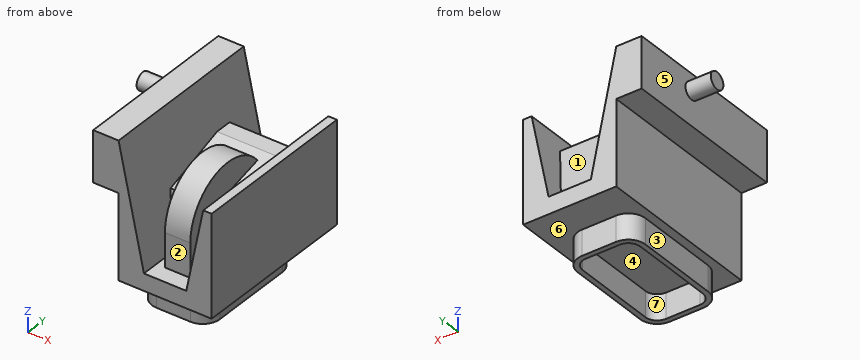
from build123d import *

# Parameters (mm, degrees)
F1_DEPTH      = 100
F4_DEPTH      = 20.5
F4_DEPTH_BACK = 21.0714285714
F6_DEPTH      = 7.5
F6_DEPTH_BACK = 7.5
F7_W          = 15
F7_H          = 30
F8_DEPTH      = 100
F9_R          = 5
F10_DEPTH     = 15
F11_W         = 40
F11_H         = 70
F12_DEPTH     = 15
F13_R         = 10
F15_DEPTH     = 15


with BuildPart() as f1:
    # F0 (on Front) → F1 (new body)
    with BuildSketch(Plane.XZ):
        Polygon((15, 10), (0, 80), (0, 0), (55, 0), (55, 60), (50, 60), (40, 10), align=None)
    extrude(amount=-F1_DEPTH)

    # F3 (on offset) → F4 (join, two sides)
    with BuildSketch(Plane.YZ.offset(27.5)) as f4_sk:
        Polygon((30, 40), (21.9615242271, 10), (90, 10), (80, 50), (70, 50), align=None)
    extrude(amount=F4_DEPTH)
    extrude(f4_sk.sketch, amount=-F4_DEPTH_BACK)

    # F5 (on offset) → F6 (join, two sides)
    with BuildSketch(Plane.YZ.offset(27.5)) as f6_sk:
        with BuildLine():
            Line((10, 0), (40, 0))
            ThreePointArc((40, 0), (61.2132034356, 51.2132034356), (10, 30))
            Line((10, 30), (10, 0))
        make_face()
    extrude(amount=F6_DEPTH)
    extrude(f6_sk.sketch, amount=-F6_DEPTH_BACK)

    # F7 (on face) → F8 (join)
    with BuildSketch(Plane.XZ):
        with Locations((-7.5, 65)):
            Rectangle(F7_W, F7_H)
    extrude(amount=-F8_DEPTH)

    # F9 (on face) → F10 (join)
    with BuildSketch(Plane(origin=(-15, 0, 0), x_dir=(0, -1, 0), z_dir=(-1, 0, 0))):
        with Locations((-60, 70)):
            Circle(F9_R)
    extrude(amount=F10_DEPTH)

    # F11 (on face) → F12 (join)
    with BuildSketch(Plane(origin=(0, 0, 0), x_dir=(1, 0, 0), z_dir=(0, 0, -1))):
        with Locations((25, -45)):
            Rectangle(F11_W, F11_H)
    extrude(amount=F12_DEPTH)

    # F13
    f13_edges = [f1.edges().sort_by_distance(p)[0] for p in [
        (45, 10, -7.5),
        (5, 10, -7.5),
        (45, 80, -7.5),
        (5, 80, -7.5),
    ]]
    fillet(f13_edges, radius=F13_R)

    # F14 (on face) → F15 (cut)
    with BuildSketch(Plane(origin=(0, 0, -15), x_dir=(1, 0, 0), z_dir=(0, 0, -1))):
        with BuildLine():
            Line((8, -20), (8, -70))
            ThreePointArc((8, -70), (10.0502525317, -74.9497474683), (15, -77))
            Line((15, -77), (35, -77))
            ThreePointArc((35, -77), (39.9497474683, -74.9497474683), (42, -70))
            Line((42, -70), (42, -20))
            ThreePointArc((42, -20), (39.9497474683, -15.0502525317), (35, -13))
            Line((35, -13), (15, -13))
            ThreePointArc((15, -13), (10.0502525317, -15.0502525317), (8, -20))
        make_face()
    extrude(amount=-F15_DEPTH, mode=Mode.SUBTRACT)


solid = f1.part
The model under review builds one solid part; all positions refer to its coordinate system, in mm. Face numbers are marked on the shaded views. A direction names the side the tool comes from. Round coordinates to 2 decimals unless told otherwise and drop trailing zeros. Order: outer loops, then holes, each group sorted by start corner. A loop starts at its lowest first (then second) coordinate and runs counter-clockwise, first axis right, second up. Notation, with made-up numbers: (70, 72.5) -> (83, 72.5) arc R10 ccw to (83, 77.5) -> close; hole circle Ø7 at (-24.75, -7). An arc over 180 degrees is marked (long way). Return JSON: item names as keys, results as strings.
1. Insertion check: P1, Ø15, axis at y = 49, z = 19, coming from the -X side; P2, Ø16.5, axis at x = 27, y = 52, coming from the -Z side; P3, Ø16.5, axis at x = 25.5, z = -8.5, coming from the +Y side. Each pin has a flat end and moves straight along its axis. Give the tip position at first contact, or say it passes through.
Answer block:
{"P1": "stops at x = 0", "P2": "stops at z = 0", "P3": "stops at y = 80"}
2. For the marked faces 1, 2, 3 and 4, list the 3-axis set-ups (+Z, -Z, +X, -X, +Y, -Y) from which the entire face can be reached by the end or side of a thin tool; tool diameter is ignored.
Answer block:
{"face 1": "+Z, +Y", "face 2": "+Z, -Y", "face 3": "-Z, -X, +Y, -Y", "face 4": "-Z"}
3. Take a section at A-A (z = 52.5). Write out the cut boundary in (x, y).
Answer block:
{"outline": "(-15, 0) -> (5.89, 0) -> (5.89, 100) -> (-15, 100) -> close; (20, 20.16) -> (35, 20.16) -> (35, 59.84) -> (20, 59.84) -> close; (48.5, 0) -> (55, 0) -> (55, 100) -> (48.5, 100) -> close"}
4. Take a section at D-D (x = -3). Write out the cut boundary in (y, z), then the cut area to 3 significant figures.
Answer block:
{"outline": "(0, 50) -> (100, 50) -> (100, 80) -> (0, 80) -> close", "area": "3,000 mm²"}
5. The part is to be moulded in two halves that separate along X. For the marked faces 5, 6 and 7, say which applies: +X half, -X half, draft (parallel to the pull), parting line (faces both ways), or undercut.
Answer block:
{"face 5": "-X half", "face 6": "draft", "face 7": "undercut"}
6. Take a section at B-B (y = 25.5). Write out the cut boundary in (x, z).
Answer block:
{"outline": "(-15, 50) -> (0, 50) -> (0, 0) -> (5, 0) -> (5, -15) -> (8, -15) -> (8, 0) -> (42, 0) -> (42, -15) -> (45, -15) -> (45, 0) -> (55, 0) -> (55, 60) -> (50, 60) -> (42.64, 23.21) -> (35, 23.21) -> (35, 56.26) -> (20, 56.26) -> (20, 23.21) -> (12.17, 23.21) -> (0, 80) -> (-15, 80) -> close"}
7. Take a section at C-C (z = 41.5). Write out the cut boundary in (x, y) (3 decimals).
Answer block:
{"outline": "(0, 0) -> (8.25, 0) -> (8.25, 36) -> (20, 36) -> (20, 12.292) -> (35, 12.292) -> (35, 36) -> (46.3, 36) -> (46.3, 0) -> (55, 0) -> (55, 100) -> (46.3, 100) -> (46.3, 82.125) -> (8.25, 82.125) -> (8.25, 100) -> (0, 100) -> close"}
8. For L1, parallel to X at y = 59, z = -3.5; L2, parallel to Z at x = 15, y = 72.5; L3, parallel to Z at x = 27.5, y = 77.5, list the stretches that pass through material, from the lowest coordinate up. Write a range as [from, to].
Answer block:
{"L1": "x = [5, 8], [42, 45]", "L2": "z = [0, 50]", "L3": "z = [-15, 50]"}
